Check sheet for the modelled part. Datum: model origin and axes. Units: mm. A direction names the side the tool comes from. Give positions to 0.01 mm unless a question says otherwise; leave off trailing zeros. Loops run counter-clockwise (first coordinate to the right, second up) from the corner with the lowest first, then second, coordinate; pieces in that order, holes last. Notation, with made-up numbers: (27.5, 80.25) - (81.5, 80.25) arc R14 ccw to (81.5, 90.25) - close; hole circle Ø2 at (-34, 26). An arc over 180 degrees is marked (long way). Use CSV: the item, a comma, the result in double quotes.
from build123d import *

# Parameters (mm, degrees)
F1_DEPTH  = 47
F3_DEPTH  = 45
F5_DEPTH  = 2
F7_DEPTH  = 1
F8_R      = 1
F9_W      = 5
F9_H      = 10
F9_H_2    = 4
F9_H_3    = 2
F10_DEPTH = 1
F13_DEPTH = 3
F15_DEPTH = 1
F17_DEPTH = 1


with BuildPart() as f1:
    # F0 (on Front) → F1 (new body)
    with BuildSketch(Plane.XZ):
        with BuildLine():
            Line((-3.2912763482, 0), (3.2912763482, 0))
            ThreePointArc((3.2912763482, 0), (0, 30.95), (-3.2912763482, 0))
        make_face()
    extrude(amount=F1_DEPTH)

    # F2 (on face) → F3 (cut)
    with BuildSketch(Plane(origin=(0, 0, 0), x_dir=(-1, 0, 0), z_dir=(0, 1, 0))):
        with BuildLine():
            Line((0, 25.95), (0, 30.95))
            ThreePointArc((0, 30.95), (-12.5454312905, 24.6559956037), (-15, 10.8365372187))
            Line((-15, 10.8365372187), (-9, 10.8365372187))
            Line((-9, 10.8365372187), (-9, 5.95))
            Line((-9, 5.95), (7, 5.95))
            Line((7, 5.95), (7, 25.95))
            Line((7, 25.95), (0, 25.95))
        make_face()
    extrude(amount=-F3_DEPTH, mode=Mode.SUBTRACT)

    # F4 (on face) → F5 (join)
    with BuildSketch(Plane(origin=(0, -45, 0), x_dir=(-1, 0, 0), z_dir=(0, 1, 0))):
        Polygon((-9, 25.95), (-9, 10.8365372187), (-9, 5.95), (7, 5.95), (7, 25.95), (0, 25.95), align=None)
    extrude(amount=F5_DEPTH)

    # F6 (on face) → F7 (cut)
    with BuildSketch(Plane(origin=(0, -43, 0), x_dir=(-1, 0, 0), z_dir=(0, 1, 0))):
        Polygon((0, 23.95), (-7, 23.95), (-7, 7.95), (5, 7.95), (5, 23.95), align=None)
    extrude(amount=-F7_DEPTH, mode=Mode.SUBTRACT)

    # F8
    f8_edges = [f1.edges().sort_by_distance(p)[0] for p in [
        (7, -43.5, 23.95),
        (-5, -43.5, 23.95),
        (7, -43.5, 7.95),
        (-5, -43.5, 7.95),
    ]]
    fillet(f8_edges, radius=F8_R)

    # F9 (on face) → F10 (join)
    with BuildSketch(Plane.YZ.offset(-7)):
        with Locations((-39.5, 10.95)):
            Rectangle(F9_W, F9_H)
        with Locations((-39.5, 18.95)):
            Rectangle(F9_W, F9_H_2)
        with Locations((-39.5, 22.95)):
            Rectangle(F9_W, F9_H_3)
        with Locations((-32.5, 22.95)):
            Rectangle(F9_W, F9_H_3)
        with Locations((-32.5, 18.95)):
            Rectangle(F9_W, F9_H_2)
        with Locations((-32.5, 10.95)):
            Rectangle(F9_W, F9_H)
        with Locations((-25.5, 22.95)):
            Rectangle(F9_W, F9_H_3)
        with Locations((-25.5, 18.95)):
            Rectangle(F9_W, F9_H_2)
        with Locations((-25.5, 10.95)):
            Rectangle(F9_W, F9_H)
        with Locations((-18.5, 22.95)):
            Rectangle(F9_W, F9_H_3)
        with Locations((-18.5, 18.95)):
            Rectangle(F9_W, F9_H_2)
        with Locations((-18.5, 10.95)):
            Rectangle(F9_W, F9_H)
        with Locations((-4.5, 22.95)):
            Rectangle(F9_W, F9_H_3)
        with Locations((-4.5, 18.95)):
            Rectangle(F9_W, F9_H_2)
        with Locations((-4.5, 10.95)):
            Rectangle(F9_W, F9_H)
    extrude(amount=F10_DEPTH)

    # F12 (on offset) → F13 (join)
    with BuildSketch(Plane(origin=(0, -13, 0), x_dir=(-1, 0, 0), z_dir=(0, 1, 0))):
        Polygon((7, 25.95), (0, 25.95), (-9, 25.95), (-9, 10.8365372187), (-9, 5.95), (7, 5.95), align=None)
    extrude(amount=F13_DEPTH)

    # F14 (on face) → F15 (cut)
    with BuildSketch(Plane(origin=(0, -10, 0), x_dir=(-1, 0, 0), z_dir=(0, 1, 0))):
        with BuildLine():
            ThreePointArc((4, 7.95), (4.7071067812, 8.2428932188), (5, 8.95))
            Line((5, 8.95), (5, 22.95))
            ThreePointArc((5, 22.95), (4.7071067812, 23.6571067812), (4, 23.95))
            Line((4, 23.95), (-6, 23.95))
            ThreePointArc((-6, 23.95), (-6.7071067812, 23.6571067812), (-7, 22.95))
            Line((-7, 22.95), (-7, 8.95))
            ThreePointArc((-7, 8.95), (-6.7071067812, 8.2428932188), (-6, 7.95))
            Line((-6, 7.95), (4, 7.95))
        make_face()
    extrude(amount=-F15_DEPTH, mode=Mode.SUBTRACT)

    # F16 (on face) → F17 (cut)
    with BuildSketch(Plane.XZ.offset(13)):
        with BuildLine():
            Line((-4, 7.95), (6, 7.95))
            ThreePointArc((6, 7.95), (6.7071067812, 8.2428932188), (7, 8.95))
            Line((7, 8.95), (7, 22.95))
            ThreePointArc((7, 22.95), (6.7071067812, 23.6571067812), (6, 23.95))
            Line((6, 23.95), (-4, 23.95))
            ThreePointArc((-4, 23.95), (-4.7071067812, 23.6571067812), (-5, 22.95))
            Line((-5, 22.95), (-5, 8.95))
            ThreePointArc((-5, 8.95), (-4.7071067812, 8.2428932188), (-4, 7.95))
        make_face()
    extrude(amount=-F17_DEPTH, mode=Mode.SUBTRACT)


solid = f1.part
1. Go/stop test with flat-tipped pins: pin 1 Ø4 at (x, y) = (-9.5, -8.5) entering from -Z; pin 2 Ø8 at (y, z) = (-37.5, 22) entering from -X; pin 3 Ø0.6 at (x, y) = (5.5, -44) entering from +Z. Record where each tip stops, or that it passes through.
Completed:
pin 1,"stops at z = 1.56"
pin 2,"stops at x = -15.42"
pin 3,"stops at z = 25.95"
2. Sectioned sample at C-C, the plane y = -3. Record the boundary of the cut face in (x, z).
Completed:
outline,"(-7, 15.95) - (-7, 16.95) - (-6, 16.95) - (-6, 20.95) - (-7, 20.95) - (-7, 21.95) - (-6, 21.95) - (-6, 23.95) - (-7, 23.95) - (-7, 25.95) - (0, 25.95) - (0, 30.95) arc R15.65 ccw to (-3.29, 0) - (3.29, 0) arc R15.65 ccw to (15, 10.84) - (9, 10.84) - (9, 5.95) - (-6, 5.95) - (-6, 15.95) - close"
3. Sectioned sample at B-B, the plane x = 2.5. Record the boundary of the cut face in (y, z).
Completed:
outline,"(-47, 0) - (0, 0) - (0, 5.95) - (-10, 5.95) - (-10, 7.95) - (-11, 7.95) - (-11, 23.95) - (-10, 23.95) - (-10, 25.95) - (-13, 25.95) - (-13, 23.95) - (-12, 23.95) - (-12, 7.95) - (-13, 7.95) - (-13, 5.95) - (-43, 5.95) - (-43, 7.95) - (-44, 7.95) - (-44, 23.95) - (-43, 23.95) - (-43, 25.95) - (-45, 25.95) - (-45, 30.75) - (-47, 30.75) - close"
4. Release check for a two-part mould opening along X. For faces 4 (the face through (-6, -5, 19)), 5 (the face through (-6.5, -4.5, 20.95)), 6 (the face through (6.715, -43.507, 23.649)) record: released by +X, released by -X, zero draft, split by the parting line, or undercut.
Completed:
face 4,"released by +X"
face 5,"zero draft"
face 6,"undercut"
5. Set-up check for faces 1 (the face through (-5, -43.5, 15.9)), 2 (the face through (12, -22, 10.837)), 3 (the face through (-6.5, -42, 18.9)): record each of +Z, -Z, +X, -X, +Y, -Y from which the full face is reachable in a straight line by a thin tool's end or side.
Completed:
face 1,"none"
face 2,"+Z, +X, +Y"
face 3,"+X"
6. Sectioned sample at D-D, the plane z = 27.5. Record the boundary of the cut face in (x, y).
Completed:
outline,"(-9.8, -47) - (9.8, -47) - (9.8, -45) - (0, -45) - (0, 0) - (-9.8, 0) - close"
7. Scan lines: line 1 along Y through (x, z) = (-3.5, 8); line 2 along Y through (x, z) = (0.5, 7); line 3 along Y through (x, z) = (2, 27.5). Record each from-to range of solid material in increasing order.
Completed:
line 1,"y = -47 to -44, -12 to -11"
line 2,"y = -47 to -43, -13 to -10"
line 3,"y = -47 to -45"
8. Sectioned sample at A-A, the plane y = -9. Record the boundary of the cut face in (x, z), and give its area (3 significant figures).
Completed:
outline,"(-7, 5.95) - (-7, 25.95) - (0, 25.95) - (0, 30.95) arc R15.65 ccw to (-3.29, 0) - (3.29, 0) arc R15.65 ccw to (15, 10.84) - (9, 10.84) - (9, 5.95) - close"
area,"323 mm²"
